Read the model definition and answer for the solid it produces. Units are mm, in the model's axes. Face numbers are marked on the shaded views. A direction names the side the tool comes from. Coordinates: 2 decimals unless noted, no trailing zeros. Use CSV: the item, a comma, the result in double quotes.
```python
from build123d import *

# Parameters (mm, degrees)
SKETCH1_R           = 5
SKETCH1_R_2         = 1.8
BOSS_EXTRUDE1_DEPTH = 10
CHAMFER1_SIZE       = 0.5
CUT_EXTRUDE2_DEPTH  = 2.5
CHAMFER2_SIZE       = 0.5
SKETCH4_R           = 1.8
CUT_EXTRUDE3_DEPTH  = 10
CHAMFER3_SIZE       = 0.5
CHAMFER3_SIZE_2     = 0.923879533
CHAMFER3_SIZE_3     = 0.552958444
SKETCH7_R           = 10.975
SKETCH7_R_2         = 4
BOSS_EXTRUDE2_DEPTH = 5.18
SKETCH8_R           = 8.5125
CUT_EXTRUDE6_DEPTH  = 11.18
SKETCH9_R           = 9.5125
CUT_EXTRUDE8_DEPTH  = 6.32
CHAMFER4_SIZE       = 0.25


with BuildPart() as part:
    # Sketch1 → Boss-Extrude1 (new body)
    with BuildSketch(Plane.XY):
        with BuildLine():
            Line((-40.746699048, 8.183561953), (-33.214821075, -10))
            Line((-33.214821075, -10), (-9.797958971, -10))
            ThreePointArc((-9.797958971, -10), (0, -14), (9.797958971, -10))
            Line((9.797958971, -10), (19.5, -10))
            Line((19.5, -10), (19.5, -3.981225471))
            ThreePointArc((19.5, -3.981225471), (20, 4.0125), (20.5, -3.981225471))
            Line((20.5, -3.981225471), (20.5, -10))
            Line((20.5, -10), (33.214821075, -10))
            Line((33.214821075, -10), (40.746699048, 8.183561953))
            ThreePointArc((40.746699048, 8.183561953), (0, 18.25), (-40.746699048, 8.183561953))
        make_face()
        Circle(SKETCH1_R, mode=Mode.SUBTRACT)
        with Locations((-32.052211881, 8.130884627)):
            Circle(SKETCH1_R_2, mode=Mode.SUBTRACT)
        with Locations(Location((32.052211881, 8.130884627, 0), (0, 0, 180))):
            Circle(SKETCH1_R_2, mode=Mode.SUBTRACT)
        with Locations((-22, 10)):
            Circle(SKETCH1_R_2, mode=Mode.SUBTRACT)
        with Locations(Location((22, 10, 0), (0, 0, 180))):
            Circle(SKETCH1_R_2, mode=Mode.SUBTRACT)
        Polygon((-25.988511975, 6.5901118), (-35.250404289, 2.75371039), (-31.414002879, -6.508181923), (-22.152110566, -2.671780514), align=None, mode=Mode.SUBTRACT)
    extrude(amount=BOSS_EXTRUDE1_DEPTH)

    # Chamfer1
    chamfer1_edges = [part.edges().sort_by_distance(p)[0] for p in [
        (20, 4.0125, 0),
        (-24.070311271, 1.959165643, 0),
        (-30.619458132, 4.671911095, 0),
        (-33.332203584, -1.877235766, 0),
        (-26.783056723, -4.589981218, 0),
    ]]
    chamfer(chamfer1_edges, length=CHAMFER1_SIZE)

    # Sketch3 → Cut-Extrude2 (cut)
    with BuildSketch(Plane.XY.offset(3.75)):
        Polygon((-37.076762037, 12.944469155), (-33.567560961, 4.472508325), (-28.393835579, 6.615535546), (-31.903036655, 15.087496376), align=None)
        Polygon((37.076762037, 12.944469155), (33.567560961, 4.472508325), (28.393835579, 6.615535546), (31.903036655, 15.087496376), align=None)
    extrude(amount=CUT_EXTRUDE2_DEPTH, mode=Mode.SUBTRACT)

    # Chamfer2
    chamfer2_edges = [part.edges().sort_by_distance(p)[0] for p in [
        (14.648979486, -10, 0),
        (0, -14, 0),
        (-21.506390023, -10, 0),
        (-36.980760062, -0.908219024, 0),
        (0, 18.25, 0),
        (36.980760062, -0.908219024, 0),
        (26.857410538, -10, 0),
    ]]
    chamfer(chamfer2_edges, length=CHAMFER2_SIZE)

    # Sketch4 → Cut-Extrude3 (cut)
    with BuildSketch(Plane(origin=(-29.114518455, -12.059628406, 0), x_dir=(0, 0, -1), z_dir=(0.9238795325112882, 0.38268343236508634, 0))):
        with Locations(Location((-5.25, 11.021342374, 0), (0, 0, 90))):
            Circle(SKETCH4_R)
    extrude(amount=-CUT_EXTRUDE3_DEPTH, mode=Mode.SUBTRACT)

    # Chamfer3
    # the kernel refuses this chamfer: 0.923879533, 0.552958444, 0.5 mm, written as the material it takes off along each edge
    with BuildSketch(Plane(origin=(40.746699048, 8.183561953, -0.920037939), x_dir=(-0.38268343236508906, -0.923879532511287, 0), z_dir=(0, 0, 1))) as chamfer3_piece_1:
        with BuildLine():
            Line((CHAMFER3_SIZE, 0), (-0.048717445, -0.548717445))
            ThreePointArc((-0.048717445, -0.548717445), (-0.025540103, -0.282767493), (0, 0))
            Line((0, 0), (CHAMFER3_SIZE, 0))
        make_face()
    extrude(amount=12.340075878, mode=Mode.SUBTRACT)
    with BuildSketch(Plane(origin=(33.214821075, -10, -1.895315111), x_dir=(-1, 0, 0), z_dir=(0, 0, 1)), Plane(origin=(-33.214821075, -10, -1.895315111), x_dir=(-0.38268343236508656, 0.9238795325112881, 0), z_dir=(0, 0, 1))) as chamfer3_piece_2:
        Polygon((CHAMFER3_SIZE, 0), (-CHAMFER3_SIZE_2 * 0.382683432163, -CHAMFER3_SIZE_2 * 0.923879532023), (0, 0), align=None)
    extrude(amount=14.290630221, mode=Mode.SUBTRACT)
    with BuildSketch(Plane(origin=(-40.746699048, 8.183561953, -0.925350902), x_dir=(0.38268343236508684, -0.9238795325112881, 0), z_dir=(0, 0, 1))) as chamfer3_piece_3:
        with BuildLine():
            Line((CHAMFER3_SIZE_3, 0), (-0.04424113, 0.496614821))
            ThreePointArc((-0.04424113, 0.496614821), (-0.0231658, 0.256042208), (0, 0))
            Line((0, 0), (CHAMFER3_SIZE_3, 0))
        make_face()
    extrude(amount=12.350701805, mode=Mode.SUBTRACT)

    # Sketch7 → Boss-Extrude2 (add)
    with BuildSketch(Plane.XY.offset(10)):
        Circle(SKETCH7_R)
        Circle(SKETCH7_R_2, mode=Mode.SUBTRACT)
    extrude(amount=BOSS_EXTRUDE2_DEPTH)

    # Sketch8 → Cut-Extrude6 (cut)
    with BuildSketch(Plane.XY):
        with Locations(Location((0, 0, 0), (0, 0, 180))):
            Circle(SKETCH8_R)
    extrude(amount=CUT_EXTRUDE6_DEPTH, mode=Mode.SUBTRACT)

    # Sketch9 → Cut-Extrude8 (cut)
    with BuildSketch(Plane.XY):
        with Locations(Location((0, 0, 0), (0, 0, 180))):
            Circle(SKETCH9_R)
    extrude(amount=CUT_EXTRUDE8_DEPTH, mode=Mode.SUBTRACT)

    # Chamfer4
    chamfer4_edges = [part.edges().sort_by_distance(p)[0] for p in [
        (-10.975, 0, 15.18),
        (-4, 0, 15.18),
        (8.5125, 0, 6.32),
    ]]
    chamfer(chamfer4_edges, length=CHAMFER4_SIZE)


solid = part.part
```
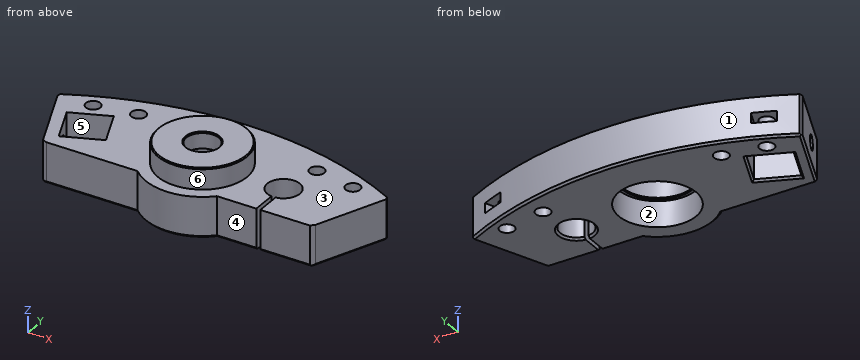
Item 1: The mould has two halves that part along X. Classify the marked faces 1, 2 and 3: +X half, -X half, draft (parallel to the pull), parting line (faces both ways), or undercut.
Return value:
face 1,"parting line"
face 2,"undercut"
face 3,"draft"
Item 2: Straight lines are drawn through the part: line 1 along Y through (x, z) = (22, 7.75); line 2 along Y through (x, z) = (0, 12.65) (3 decimals); line 3 along X through (y, z) = (-8.5, 3). For each, find the intervals that lie inside material, in ascending order.
Return value:
line 1,"y = -10 to -3.48, 3.48 to 8.2, 11.8 to 15.44"
line 2,"y = -10.975 to -4, 4 to 10.975"
line 3,"x = -33.84 to -4.27, 4.27 to 19.5, 20.5 to 33.84"
Item 3: Find section B-B, the plane z = 1.75. Give the number of separate pieces and of enclosed holes in the cut face, then the cut area to 3 significant figures.
Return value:
separate pieces,"1"
enclosed holes,"6"
area,"1,470 mm^2"
Item 4: A tool of negligible diameter and unlimited length cuts with its end or side. For the marked faces 4, 5 and 6, from which of +Z, -Z, +X, -X, +Y, -Y can it reach the whole face along a straight path? Write none if from no direction.
Return value:
face 4,"+Z, -Z, +X, -Y"
face 5,"+Z, -Z"
face 6,"+Z"
Item 5: Each of these flat-tipped pins is pushed along its axis until it touches: P1, Ø6, axis at x = 32.05, y = 8.13, coming from the +Z side; P2, Ø3, axis at x = -17.5, z = 3.5, coming from the -Y side; P3, Ø3, axis at y = -7, z = 7, coming from the +X side. Where does it stop, or does it pass through?
Return value:
P1,"stops at z = 10"
P2,"stops at y = -10"
P3,"stops at x = 35.08"
